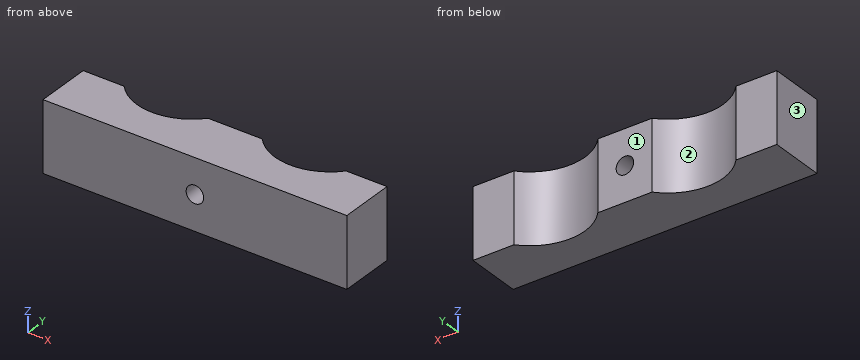
from build123d import *

# Parameters (mm, degrees)
SKETCH4_W           = 55
SKETCH4_H           = 10
BOSS_EXTRUDE1_DEPTH = 12.7
SKETCH5_R           = 10
CUT_EXTRUDE1_DEPTH  = 58.326172033
SKETCH8_R           = 1.5875
CUT_EXTRUDE3_DEPTH  = 58.326172033


with BuildPart() as part:
    # Sketch4 → Boss-Extrude1 (new body)
    with BuildSketch(Plane.XY):
        with Locations((27.5, 5)):
            Rectangle(SKETCH4_W, SKETCH4_H)
    extrude(amount=BOSS_EXTRUDE1_DEPTH)

    # Sketch5 → Cut-Extrude1 (cut, through all)
    with BuildSketch(Plane.XY.offset(12.7)):
        with Locations((15, 16.5)):
            Circle(SKETCH5_R)
        with Locations((40, 16.5)):
            Circle(SKETCH5_R)
    extrude(amount=-CUT_EXTRUDE1_DEPTH, mode=Mode.SUBTRACT)

    # Sketch8 → Cut-Extrude3 (cut, through all)
    with BuildSketch(Plane(origin=(0, 10, 0), x_dir=(1, 0, 0), z_dir=(0, 1, 0))):
        with Locations(Location((27.5, -6.35, 0), (0, 0, 270))):
            Circle(SKETCH8_R)
    extrude(amount=-CUT_EXTRUDE3_DEPTH, mode=Mode.SUBTRACT)


solid = part.part
Could you check a few things on this model? Use its own coordinates, in mm. Face numbers are marked on the shaded views. Round coordinates to 2 decimals unless told otherwise and drop trailing zeros. Loops run counter-clockwise (first coordinate to the right, second up) from the corner with the lowest first, then second, coordinate; pieces in that order, holes last. Notation, with made-up numbers: (22.25, 66) - (36.25, 66) arc R10 ccw to (36.25, 76) - close; hole circle Ø9 at (-4, -33). An arc over 180 degrees is marked (long way). Write item = value, one per line.
1) Imagine slicing it at A-A (x = 27.5). Please give me the cut outline in (y, z), and give its area (4 significant figures).
Computed:
outline = (0, 0) - (10, 0) - (10, 4.76) - (0, 4.76) - close; (0, 7.94) - (10, 7.94) - (10, 12.7) - (0, 12.7) - close
area = 95.25 mm2
2) I'm going to push a flat-ended pin straight in: P1, Ø1.5, axis at x = 36, z = 1.5, coming from the +Y side. Where does the tip first touch, or does it pass through?
Computed:
P1 = 7.7
3) Imagine slicing it at D-D (x = 45). Please give me the cut outline in (y, z).
Computed:
outline = (0, 0) - (7.84, 0) - (7.84, 12.7) - (0, 12.7) - close
4) Imagine slicing it at C-C (z = 1.75). Please give me the cut outline in (x, y).
Computed:
outline = (0, 0) - (55, 0) - (55, 10) - (47.6, 10) arc R10 cw to (32.4, 10) - (22.6, 10) arc R10 cw to (7.4, 10) - (0, 10) - close
5) If we mould it in two halves opening along X, with no side actions, what happens to the marked faces 1, 2 and 3? For each: pulls with the +X half, pulls with the -X half, needs draft (parallel to the pull), parting line crosses it, or undercut.
Computed:
face_1 = needs draft
face_2 = undercut
face_3 = pulls with the -X half
6) I need wall thicknesses on line 1 along X through (y, z) = (2.75, 6.35); line 2 along X through (y, z) = (8, 8.5); line 3 along X through (y, z) = (7.25, 6.35). Which ranges of each line are inside material? Lowest first, please. Write a range as from..to.
Computed:
line_1 = 0..25.91, 29.09..55
line_2 = 0..9.73, 20.27..34.73, 45.27..55
line_3 = 0..11.2, 18.8..25.91, 29.09..36.2, 43.8..55
7) Imagine slicing it at B-B (z = 6.35). Please give me the cut outline in (x, y), and give its area (3 significant figures).
Computed:
outline = (0, 0) - (25.91, 0) - (25.91, 10) - (22.6, 10) arc R10 cw to (7.4, 10) - (0, 10) - close; (29.09, 0) - (55, 0) - (55, 10) - (47.6, 10) arc R10 cw to (32.4, 10) - (29.09, 10) - close
area = 444 mm2
